```python
from build123d import *

# Parameters (mm, degrees)
SKETCH001_W     = 150
SKETCH001_H     = 24.5
PAD_DEPTH       = 60
SKETCH_W        = 18
SKETCH_H        = 4
PAD001_DEPTH    = 8
SKETCH002_W     = 15.4
SKETCH002_H     = 6
SKETCH002_W_2   = 17.726488
POCKET_DEPTH    = 2
SKETCH003_W     = 15.4
SKETCH003_H     = 6
SKETCH003_W_2   = 17.726488
POCKET001_DEPTH = 2
SKETCH004_W     = 70
SKETCH004_H     = 8
POCKET002_DEPTH = 60.001
FILLET_R        = 3.8


with BuildPart() as part:
    # Sketch001 → Pad (new body)
    with BuildSketch(Plane.XY.offset(60)):
        with Locations((75, 12.25)):
            Rectangle(SKETCH001_W, SKETCH001_H)
    extrude(amount=PAD_DEPTH)

    # Sketch → Pad001 (new body)
    with BuildSketch(Plane.XY.offset(120)):
        with Locations((20, 5.5)):
            Rectangle(SKETCH_W, SKETCH_H)
        with Locations((20, 19.5)):
            Rectangle(SKETCH_W, SKETCH_H)
        with Locations((130, 19.5)):
            Rectangle(SKETCH_W, SKETCH_H)
        with Locations((130, 5.5)):
            Rectangle(SKETCH_W, SKETCH_H)
    extrude(amount=PAD001_DEPTH)

    # Sketch002 → Pocket (cut)
    with BuildSketch(Plane(origin=(0, 21.5, 60), x_dir=(-1, 0, 0), z_dir=(0, 1, 0))):
        with Locations((-132.7, 63)):
            Rectangle(SKETCH002_W, SKETCH002_H)
        with Locations((-22.863244, 63)):
            Rectangle(SKETCH002_W_2, SKETCH002_H)
    extrude(amount=-POCKET_DEPTH, mode=Mode.SUBTRACT)

    # Sketch003 → Pocket001 (cut)
    with BuildSketch(Plane(origin=(0, 7.5, 60), x_dir=(-1, 0, 0), z_dir=(0, 1, 0))):
        with Locations((-132.7, 63)):
            Rectangle(SKETCH003_W, SKETCH003_H)
        with Locations((-22.863244, 63)):
            Rectangle(SKETCH003_W_2, SKETCH003_H)
    extrude(amount=-POCKET001_DEPTH, mode=Mode.SUBTRACT)

    # Sketch004 → Pocket002 (cut, through all)
    with BuildSketch(Plane.XY.offset(120)):
        with Locations((75, 20.5)):
            Rectangle(SKETCH004_W, SKETCH004_H)
        with Locations((75, 4)):
            Rectangle(SKETCH004_W, SKETCH004_H)
    extrude(amount=-POCKET002_DEPTH, mode=Mode.SUBTRACT)

    # Fillet
    fillet_edges = [part.edges().sort_by_distance(p)[0] for p in [
        (150, 0, 90),
        (110, 0, 90),
        (110, 8, 90),
        (110, 16.5, 90),
        (110, 24.5, 90),
        (150, 24.5, 90),
        (0, 0, 90),
        (0, 24.5, 90),
        (40, 24.5, 90),
        (40, 0, 90),
        (40, 8, 90),
        (40, 16.5, 90),
    ]]
    fillet(fillet_edges, radius=FILLET_R)


solid = part.part
```
For this review, take the finished solid that the model builds, in its own axes (mm). A direction names the side the tool comes from. Round coordinates to 2 decimals unless told otherwise and drop trailing zeros. Write each loop counter-clockwise with the first axis right and the second up, starting at its lowest first coordinate (ties: lowest second). Pieces come first, ordered by that corner, then holes.
1) Take a section at D-D on x = 117. Give the boundary of the cut face in (y, z), then the cut area to 3 significant figures.
Answer below:
outline: (0, 60) - (24.5, 60) - (24.5, 120) - (0, 120) - close
area: 1,470 mm2
2) Take a section at B-B on z = 98.5. Give the boundary of the cut face in (x, y), then the cut area to 3 significant figures.
Answer below:
outline: (0, 3.8) arc R3.8 ccw to (3.8, 0) - (36.2, 0) arc R3.8 ccw to (40, 3.8) - (40, 4.2) arc R3.8 cw to (43.8, 8) - (106.2, 8) arc R3.8 cw to (110, 4.2) - (110, 3.8) arc R3.8 ccw to (113.8, 0) - (146.2, 0) arc R3.8 ccw to (150, 3.8) - (150, 20.7) arc R3.8 ccw to (146.2, 24.5) - (113.8, 24.5) arc R3.8 ccw to (110, 20.7) - (110, 20.3) arc R3.8 cw to (106.2, 16.5) - (43.8, 16.5) arc R3.8 cw to (40, 20.3) - (40, 20.7) arc R3.8 ccw to (36.2, 24.5) - (3.8, 24.5) arc R3.8 ccw to (0, 20.7) - close
area: 2,540 mm2
3) Machinability: for faces 5 (the face through (29, 5, 125)), 6 (the face through (130, 17.5, 124)), 7 (the face through (130, 3.5, 124)), 8 (the face through (22, 5.5, 123)), which of the approach directions +Z, -Z, +X, -X, +Y, -Y give a long, thin tool a straight path to every point of the face, cutting with its end or side? Answer none if there is none.
Answer below:
face 5: +Z, +Y, -Y
face 6: +Z, +X, -X
face 7: +Z, +X, -X, -Y
face 8: none
4) Mouldability with a two-part tool opening along X and no side actions: class faces 1 (the face through (121, 5, 124)), 2 (the face through (130, 20, 128)), 3 (the face through (11, 19, 124)), 4 (the face through (139, 19, 125)) as +X half, -X half, draft (parallel to the pull), parting line (faces both ways), or undercut.
Answer below:
face 1: undercut
face 2: draft
face 3: -X half
face 4: +X half
5) For line 1 along Z through (x, y) = (127.5, 5.75); line 2 along X through (y, z) = (4, 70.5); line 3 along Y through (x, z) = (57, 76), list the stretches that pass through material, from the lowest coordinate up.
Answer below:
line 1: z = 60 to 120, 126 to 128
line 2: x = 0 to 40, 110 to 150
line 3: y = 8 to 16.5
6) Take a section at A-A on x = 136.5. Give the boundary of the cut face in (y, z).
Answer below:
outline: (0, 60) - (24.5, 60) - (24.5, 120) - (19.5, 120) - (19.5, 126) - (21.5, 126) - (21.5, 128) - (17.5, 128) - (17.5, 120) - (5.5, 120) - (5.5, 126) - (7.5, 126) - (7.5, 128) - (3.5, 128) - (3.5, 120) - (0, 120) - close
7) Insertion check: pin 1 Ø4.5 at (y, z) = (19.5, 122.5) entering from +X; pin 2 Ø4 at (x, z) = (24.5, 123) entering from +Y; pin 3 Ø1.2 at (y, z) = (20.5, 125) entering from +X. Each pin has a flat end and moves straight along its axis. Give the tip position at first contact, or say it passes through.
Answer below:
pin 1: stops at x = 139
pin 2: stops at y = 19.5
pin 3: stops at x = 125
8) Take a section at C-C on y = 9.75. Give the boundary of the cut face in (x, z).
Answer below:
outline: (0, 60) - (150, 60) - (150, 120) - (0, 120) - close
